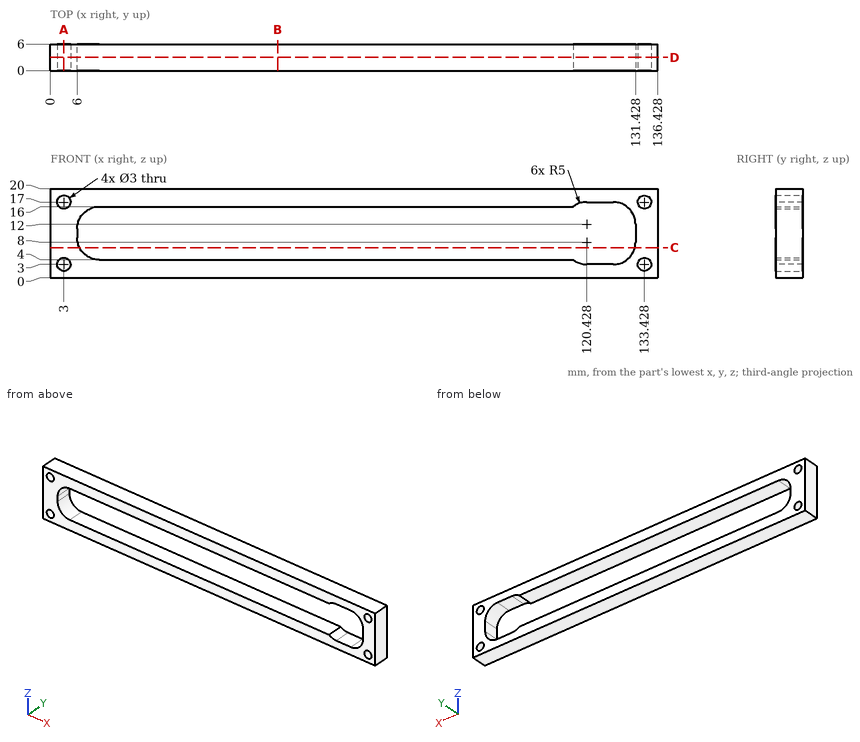
Check sheet for the drawn part. Datum: minimum x, y, z corner. Units: mm. Give positions to 0.01 mm unless a question says otherwise; leave off trailing zeros. Order: outer loops, then holes, each group sorted by start corner. A loop starts at its lowest first (then second) coordinate and runs counter-clockwise, first axis right, second up. Notation, with made-up numbers: (81.5, 67) - (100.5, 67) arc R19 cw to (100.5, 87) - close; hole circle Ø3 at (-32, 44.5). An arc over 180 degrees is marked (long way). Answer in a Markdown table with one row per item. Add a question column.
Q1. Cross-section at D-D, the plane y = 3. Enter the section's corners in (x, z).
Q2. Cross-section at B-B, the plane x = 51. Enter the section's corners in (y, z).
Q3. Gauge pin test, flat end, axial feed: pin 1 (2.5 mm diameter, centred on x = 3, z = 3, fed in from +Y). Record the tip position at first contact, or that the pin passes through.
Q4. Material ranges on probe 1 along Z at (x, y) = (3, 4.7); probe 2 along Z at (x, y) = (99.5, 3.7); probe 3 along X at (y, z) = (2.8, 2.5), recorded low to high. Write a range as from..to.
Q5. Cross-section at A-A, the plane x = 3. Enter the section's corners in (y, z).
Q6. Cross-section at C-C, the plane z = 6.75. Enter the section's corners in (x, y) (1 decimal).
Check values:
| question | item | result |
|---|---|---|
| 1 | outline | (0, 0) - (136.43, 0) - (136.43, 20) - (0, 20) - close; hole circle Ø3 at (3, 3); hole circle Ø3 at (3, 17); hole (6, 9) arc R5 ccw to (11, 4) - (117.43, 4) arc R5 ccw to (120.43, 3) - (126.43, 3) arc R5 ccw to (131.43, 8) - (131.43, 12) arc R5 ccw to (126.43, 17) - (120.43, 17) arc R5 ccw to (117.43, 16) - (11, 16) arc R5 ccw to (6, 11) - close; hole circle Ø3 at (133.43, 3); hole circle Ø3 at (133.43, 17) |
| 2 | outline | (0, 0) - (6, 0) - (6, 4) - (0, 4) - close; (0, 16) - (6, 16) - (6, 20) - (0, 20) - close |
| 3 | pin 1 | passes through |
| 4 | probe 1 | z = 0..1.5, 4.5..15.5, 18.5..20 |
| 4 | probe 2 | z = 0..4, 16..20 |
| 4 | probe 3 | x = 0..1.59, 4.41..132.01, 134.84..136.43 |
| 5 | outline | (0, 0) - (6, 0) - (6, 1.5) - (0, 1.5) - close; (0, 4.5) - (6, 4.5) - (6, 15.5) - (0, 15.5) - close; (0, 18.5) - (6, 18.5) - (6, 20) - (0, 20) - close |
| 6 | outline | (0, 0) - (6.5, 0) - (6.5, 6) - (0, 6) - close; (131.3, 0) - (136.4, 0) - (136.4, 6) - (131.3, 6) - close |
